from build123d import *

# Parameters (mm, degrees)
F1_DEPTH = 12
F2_D     = 5
F2_DEPTH = 15
F2_TIP   = 1.5021515476
F3_D     = 5
F3_DEPTH = 15
F3_TIP   = 1.5021515476
F5_D     = 4.9
F5_DEPTH = 10
F5_TIP   = 1.4721085166
F6_D     = 3.2
F6_DEPTH = 15
F6_TIP   = 0.9613769904
F7_D     = 3.2
F7_DEPTH = 15
F7_TIP   = 0.9613769904
F8_W     = 16.5
F8_H     = 6.25
F9_DEPTH = 1
F10_SIZE = 2


# Not quite as in the source:
# - a feature names something its author has since deleted; it is built from what else it names


with BuildPart() as f1:
    # F0 (on Top) → F1 (new body)
    with BuildSketch(Plane.XY):
        with BuildLine():
            Line((-19, -1.8754155822), (-19, 1.1245844178))
            Line((-19, 1.1245844178), (-15.8377223398, 1.1245844178))
            ThreePointArc((-15.8377223398, 1.1245844178), (-22.5, -0.3754155822), (-15.8377223398, -1.8754155822))
            Line((-15.8377223398, -1.8754155822), (-19, -1.8754155822))
        make_face()
        with BuildLine():
            Line((-15.8377223398, 1.1245844178), (-19, 1.1245844178))
            Line((-19, 1.1245844178), (-19, -1.8754155822))
            Line((-19, -1.8754155822), (-15.8377223398, -1.8754155822))
            ThreePointArc((-15.8377223398, -1.8754155822), (-15.5854742781, -1.144189993), (-15.5, -0.3754155822))
            ThreePointArc((-15.5, -0.3754155822), (-15.5854742781, 0.3933588286), (-15.8377223398, 1.1245844178))
        make_face()
        with BuildLine():
            Line((15.8377223398, 1.1245844178), (-15.8377223398, 1.1245844178))
            ThreePointArc((-15.8377223398, 1.1245844178), (-15.5854742781, 0.3933588286), (-15.5, -0.3754155822))
            ThreePointArc((-15.5, -0.3754155822), (-15.5854742781, -1.144189993), (-15.8377223398, -1.8754155822))
            Line((-15.8377223398, -1.8754155822), (15.8377223398, -1.8754155822))
            ThreePointArc((15.8377223398, -1.8754155822), (15.5, -0.3754155822), (15.8377223398, 1.1245844178))
        make_face()
        with BuildLine():
            ThreePointArc((22.5, -0.3754155822), (19.7687744108, 3.0391101397), (15.8377223398, 1.1245844178))
            Line((15.8377223398, 1.1245844178), (19, 1.1245844178))
            Line((19, 1.1245844178), (19, -1.8754155822))
            Line((19, -1.8754155822), (15.8377223398, -1.8754155822))
            ThreePointArc((15.8377223398, -1.8754155822), (19.7687744108, -3.7899413041), (22.5, -0.3754155822))
        make_face()
        with BuildLine():
            Line((19, 1.1245844178), (15.8377223398, 1.1245844178))
            ThreePointArc((15.8377223398, 1.1245844178), (15.5, -0.3754155822), (15.8377223398, -1.8754155822))
            Line((15.8377223398, -1.8754155822), (19, -1.8754155822))
            Line((19, -1.8754155822), (19, 1.1245844178))
        make_face()
    extrude(amount=F1_DEPTH)

    # F2
    with Locations(Plane(origin=(0, 0, 0), x_dir=(1, 0, 0), z_dir=(0, 0, -1))):
        with Locations((19, 0.3754155822)):
            Hole(F2_D / 2, depth=F2_DEPTH)
            with Locations((0, 0, -(F2_DEPTH + F2_TIP / 2))):  # 118° drill point
                Cone(0, F2_D / 2, F2_TIP, mode=Mode.SUBTRACT)

    # F3
    with Locations(Plane(origin=(0, 0, 0), x_dir=(1, 0, 0), z_dir=(0, 0, -1))):
        with Locations((-19, 0.3754155822)):
            Hole(F3_D / 2, depth=F3_DEPTH)
            with Locations((0, 0, -(F3_DEPTH + F3_TIP / 2))):  # 118° drill point
                Cone(0, F3_D / 2, F3_TIP, mode=Mode.SUBTRACT)

    # F5
    with Locations(Plane(origin=(0, 1.1245844178, 0), x_dir=(-1, 0, 0), z_dir=(0, 1, 0))):
        with Locations((0, 6)):
            Hole(F5_D / 2, depth=F5_DEPTH)
            with Locations((0, 0, -(F5_DEPTH + F5_TIP / 2))):  # 118° drill point
                Cone(0, F5_D / 2, F5_TIP, mode=Mode.SUBTRACT)

    # F6
    with Locations(Plane(origin=(0, 1.1245844178, 0), x_dir=(-1, 0, 0), z_dir=(0, 1, 0))):
        with Locations((-6, 6)):
            Hole(F6_D / 2, depth=F6_DEPTH)
            with Locations((0, 0, -(F6_DEPTH + F6_TIP / 2))):  # 118° drill point
                Cone(0, F6_D / 2, F6_TIP, mode=Mode.SUBTRACT)

    # F7
    with Locations(Plane(origin=(0, 1.1245844178, 0), x_dir=(-1, 0, 0), z_dir=(0, 1, 0))):
        with Locations((6, 6)):
            Hole(F7_D / 2, depth=F7_DEPTH)
            with Locations((0, 0, -(F7_DEPTH + F7_TIP / 2))):  # 118° drill point
                Cone(0, F7_D / 2, F7_TIP, mode=Mode.SUBTRACT)

    # F8 (on face) → F9 (cut)
    with BuildSketch(Plane(origin=(0, 1.1245844178, 0), x_dir=(-1, 0, 0), z_dir=(0, 1, 0))):
        with Locations((0, 6)):
            Rectangle(F8_W, F8_H)
    extrude(amount=-F9_DEPTH, mode=Mode.SUBTRACT)

    # F10
    f10_edges = [f1.edges().sort_by_distance(p)[0] for p in [
        (8.25, 0.624584, 9.125),
        (8.25, 0.624584, 2.875),
        (-8.25, 0.624584, 9.125),
        (-8.25, 0.624584, 2.875),
    ]]
    chamfer(f10_edges, length=F10_SIZE)


solid = f1.part
For this review, take the finished solid that the model builds, in its own axes (mm). A direction names the side the tool comes from. Give positions to 0.01 mm unless a question says otherwise; leave off trailing zeros. Loops run counter-clockwise (first coordinate to the right, second up) from the corner with the lowest first, then second, coordinate; pieces in that order, holes last.
Item 1: Insertion check: pin 1 (5.5 mm diameter, centred on x = 0, z = 6, fed in from -Y); pin 2 (5 mm diameter, centred on x = 6, z = 6, fed in from +Y); pin 3 (2 mm diameter, centred on y = 1.5, z = 6.5, fed in from +X); pin 4 (3 mm diameter, centred on x = -19, y = -0.38, fed in from +Z). Each pin has a flat end and moves straight along its axis. Give the tip position at first contact, or say it passes through.
Item 2: Draft analysis for pull direction Z (two halves, no side actions). For faces 4 (the flat face through (0, -1.875, 3)), 5 (the flat face through (0, 0, 12)), 6 (the flat face through (0, 0, 0)), 7 (the flat face through (8.25, 0.6, 6)), state which applies: +Z half, -Z half, draft (parallel to the pull), parting line (faces both ways), or undercut.
Item 3: Take a section at A-A, the plane z = 6. State the section outline as (x, y) points.
Item 4: Take a section at D-D, the plane x = 0. State the section outline as (y, z) points (3 decimals).
Item 5: For line 1 along X through (y, z) = (-0.5, 9); line 2 along X through (y, z) = (1.5, 4); line 3 along X through (y, z) = (1, 4) (3 decimals), list the stretches that pass through material, from the lowest coordinate up.
Item 6: Take a section at B-B, the plane x = -19. State the section outline as (y, z) points.
Item 7: Tool access review of faces 1 (the cylindrical face through (-5.26, -0.89, 4.58)), 2 (the flat face through (7.236, 0.632, 8.139)), 3 (the flat face through (0, 1.125, 2)): name each direction out of +Z, -Z, +X, -X, +Y, -Y from which nothing blocks a thin tool from reaching the whole face with its end or side.
Item 8: Take a section at C-C, the plane z = 10.5. State the section outline as (x, y) points.
Calculated:
1. pin 1: stops at y = -1.88
1. pin 2: stops at y = 1.12
1. pin 3: stops at x = 22.39
1. pin 4: passes through
2. face 4: draft
2. face 5: +Z half
2. face 6: -Z half
2. face 7: undercut
3. outline: (-15.84, -1.88) - (-7.6, -1.88) - (-7.6, 0.12) - (-8.25, 0.12) - (-8.25, 1.12) - (-15.84, 1.12) arc R3.5 ccw (long way) to start; (-4.4, -1.88) - (-2.45, -1.88) - (-2.45, 0.12) - (-4.4, 0.12) - close; (2.45, -1.88) - (4.4, -1.88) - (4.4, 0.12) - (2.45, 0.12) - close; (7.6, -1.88) - (15.84, -1.88) arc R3.5 ccw (long way) to (15.84, 1.12) - (8.25, 1.12) - (8.25, 0.12) - (7.6, 0.12) - close; hole circle Ø5 at (-19, -0.38); hole circle Ø5 at (19, -0.38)
4. outline: (-1.875, 0) - (1.125, 0) - (1.125, 2.875) - (0.125, 2.875) - (0.125, 3.55) - (-1.875, 3.55) - close; (-1.875, 8.45) - (0.125, 8.45) - (0.125, 9.125) - (1.125, 9.125) - (1.125, 12) - (-1.875, 12) - close
5. line 1: x = -22.5 to -21.5, -16.5 to 16.5, 21.5 to 22.5
5. line 2: x = -21.96 to -20.65, -17.35 to -16.04, 16.04 to 17.35, 20.65 to 21.96
5. line 3: x = -22.218 to -21.088, -16.912 to -7.375, 7.375 to 16.912, 21.088 to 22.218
6. outline: (-3.88, 0) - (-2.88, 0) - (-2.88, 12) - (-3.88, 12) - close; (2.12, 0) - (3.12, 0) - (3.12, 12) - (2.12, 12) - close
7. face 1: +Y, -Y
7. face 2: +Y
7. face 3: +Z, -Z, +Y
8. outline: (-15.84, -1.88) - (15.84, -1.88) arc R3.5 ccw (long way) to (15.84, 1.12) - (-15.84, 1.12) arc R3.5 ccw (long way) to start; hole circle Ø5 at (-19, -0.38); hole circle Ø5 at (19, -0.38)
